Geometry: final body of the model. Coordinates: model frame, mm. A direction names the side the tool comes from. Give positions to 0.01 mm unless a question says otherwise; leave off trailing zeros. Write each loop counter-clockwise with the first axis right and the second up, starting at its lowest first coordinate (ties: lowest second). Pieces come first, ordered by that corner, then holes. Notation, with made-up numbers: (48, 62.5) - (90, 62.5) arc R19 cw to (90, 84.5) - close; hole circle Ø3 at (4, 5). An arc over 180 degrees is marked (long way). Return JSON: item names as keys, results as strings.
from build123d import *

# Parameters (mm, degrees)
SKETCH1_R                      = 11
SKETCH1_R_2                    = 1.05
BOSS_EXTRUDE1_DEPTH            = 4
SKETCH9_R                      = 6
BOSS_EXTRUDE2_DEPTH            = 15.13
SKETCH10_OUTSIDE_W             = 31.304
SKETCH10_OUTSIDE_H             = 31.304
SKETCH10_OUTSIDE_R             = 3.5
CUT_EXTRUDE2_DEPTH             = 15
FILLET1_R                      = 4.5
FILLET2_R                      = 1
FILLET4_R                      = 4
CBORE_FOR_M2_SHCS1_D           = 2.2
CBORE_FOR_M2_SHCS1_CBORE_D     = 4.4
CBORE_FOR_M2_SHCS1_CBORE_DEPTH = 2


with BuildPart() as part:
    # Sketch1 → Boss-Extrude1 (new body)
    with BuildSketch(Plane.XY):
        Circle(SKETCH1_R)
        with Locations((0, 8)):
            Circle(SKETCH1_R_2, mode=Mode.SUBTRACT)
        with Locations((8, 0)):
            Circle(SKETCH1_R_2, mode=Mode.SUBTRACT)
        with Locations((0, -8)):
            Circle(SKETCH1_R_2, mode=Mode.SUBTRACT)
    extrude(amount=BOSS_EXTRUDE1_DEPTH)

    # Sketch9 → Boss-Extrude2 (add)
    with BuildSketch(Plane(origin=(0, 0, 0), x_dir=(-1, 0, 0), z_dir=(0, 0, -1))):
        with Locations((5, 0)):
            Circle(SKETCH9_R)
    extrude(amount=BOSS_EXTRUDE2_DEPTH)

    # Sketch10 outside → Cut-Extrude2 (cut)
    with BuildSketch(Plane(origin=(0, 0, -15.13), x_dir=(-1, 0, 0), z_dir=(0, 0, -1))):
        Rectangle(SKETCH10_OUTSIDE_W, SKETCH10_OUTSIDE_H)
        with Locations((5, 0)):
            Circle(SKETCH10_OUTSIDE_R, mode=Mode.SUBTRACT)
    extrude(amount=-CUT_EXTRUDE2_DEPTH, mode=Mode.SUBTRACT)

    # Fillet1
    # the kernel refuses this fillet: 4.5 mm, written as the material it adds along each edge
    with BuildSketch(Plane(origin=(-5, 0, 0), x_dir=(-1, 0, 0), z_dir=(0, -1, 0))) as fillet1_piece_1_section:
        with BuildLine():
            CenterArc((7.073824939, 4.5), FILLET1_R, 256.19443595, 13.80556405)
            Line((6, 0.13), (6, 0))
            Line((6, 0), (7.073824939, 0))
        make_face()
    fillet1_piece_1 = revolve(axis=Axis((-5, 0, 0), (0, 0, -1)), mode=Mode.PRIVATE)
    fillet1_piece_1 = fillet1_piece_1 & Plane(origin=(0, 0, -0.023683453), x_dir=(1, 0, 0), z_dir=(0, 0, -1)) * Cylinder(11, 29, mode=Mode.PRIVATE)
    add(fillet1_piece_1)

    # Fillet2
    fillet2_edges = [part.edges().sort_by_distance(p)[0] for p in [
        (-1.5, 0, -15.13),
    ]]
    fillet(fillet2_edges, radius=FILLET2_R)

    # Fillet4
    # the kernel refuses this fillet: 4 mm, written as the material it adds along each edge
    with BuildSketch(Plane(origin=(-5, 0, -0.13), x_dir=(-1, 0, 0), z_dir=(0, -1, 0))) as fillet4_piece_1:
        with BuildLine():
            CenterArc((7.5, 3.708099244), FILLET4_R, 180, 67.975687163)
            Line((6, 0), (5.97, -0.074161985))
            ThreePointArc((5.97, -0.074161985), (4.75, -0.08), (3.5, -0.08))
            Line((3.5, -0.08), (3.42, 0))
            Line((3.42, 0), (3.42, 3.708099244))
            Line((3.42, 3.708099244), (3.5, 3.708099244))
        make_face()
    revolve(axis=Axis((-5, 0, -0.13), (0, 0, -1)))

    # CBORE for M2 SHCS1 (through all)
    with Locations(Plane(origin=(0, 0, 0), x_dir=(-1, 0, 0), z_dir=(0, 0, -1))):
        with Locations((0, 8), (-8, 0), (0, -8)):
            CounterBoreHole(CBORE_FOR_M2_SHCS1_D / 2, CBORE_FOR_M2_SHCS1_CBORE_D / 2, CBORE_FOR_M2_SHCS1_CBORE_DEPTH)


solid = part.part
Q1. Material intervals for probe 1 along Y at (x, z) = (0, 1.45); probe 2 along Y at (x, z) = (0, 3.55); probe 3 along Z at (x, y) = (-2.75, -8.5), sorted ascending. Write a range as [from, to].
Answer key:
{"probe 1": "y = [-11, -10.2], [-5.8, 5.8], [10.2, 11]", "probe 2": "y = [-11, -9.1], [-6.9, 6.9], [9.1, 11]", "probe 3": "z = [0, 4]"}
Q2. Section query D-D, the plane x = -5. Return the cut outline in (y, z), plus the area to 3 significant figures.
Answer key:
{"outline": "(-9.8, 0) - (-7.07, 0) arc R4.5 cw to (-6, -0.13) arc R4 cw to (-3.5, -3.84) - (-3.5, -14.13) arc R1 ccw to (-2.5, -15.13) - (2.5, -15.13) arc R1 ccw to (3.5, -14.13) - (3.5, -3.84) arc R4 cw to (6, -0.13) arc R4.5 cw to (7.07, 0) - (9.8, 0) - (9.8, 4) - (-9.8, 4) - close", "area": "190 mm^2"}
Q3. Section query B-B, the plane y = 8. Return the cut outline in (x, z), plus the area to 3 significant figures.
Answer key:
{"outline": "(-7.55, 0) - (-2.2, 0) - (-2.2, 2) - (-1.1, 2) - (-1.1, 4) - (-7.55, 4) - close; (1.1, 2) - (2.2, 2) - (2.2, 0) - (7.55, 0) - (7.55, 4) - (1.1, 4) - close", "area": "47.2 mm^2"}
Q4. Set-up query: faces 4 (the flat face through (0, 0, 4)), 5 (the cylindrical face through (-1.183, 9.855, 0.986)). Return all of +Z, -Z, +X, -X, +Y, -Y with unobstructed straight access to the full face (end or side cutting, diameter ignored); none if empty.
Answer key:
{"face 4": "+Z, +X, -X, +Y, -Y", "face 5": "-Z"}
Q5. Pin query (flat end, axial travel): P1, Ø1.3, axis at x = 0, y = -8, coming from the +Z side; P2, Ø3.5, axis at x = 7, y = -0.5, coming from the -Z side; P3, Ø3.5, axis at x = 0, y = 8, coming from the +Z side; P4, Ø4, axis at x = 0, y = 8, coming from the -Z side. Return the tip coordinate at first contact, or that it passes through.
Answer key:
{"P1": "passes through", "P2": "stops at z = 0", "P3": "stops at z = 4", "P4": "stops at z = 2"}
Q6. Section query C-C, the plane z = -5.75. Return the cut outline in (x, y), plus the area to 3 significant figures.
Answer key:
{"outline": "circle Ø7 at (-5, 0)", "area": "38.5 mm^2"}
Q7. Section query A-A, the plane x = 7.5. Return the cut outline in (y, z), plus the area to 3 significant figures.
Answer key:
{"outline": "(-8.05, 0) - (-2.14, 0) - (-2.14, 2) - (-0.98, 2) - (-0.98, 4) - (-8.05, 4) - close; (0.98, 2) - (2.14, 2) - (2.14, 0) - (8.05, 0) - (8.05, 4) - (0.98, 4) - close", "area": "51.9 mm^2"}
Q8. Mould query, pull axis Y, two halves, no side actions, for faces 1 (the cylindrical face through (-8.34, 1.05, -9.06)), 2 (the flat face through (3, 0, 0)), 3 (the cylindrical face through (-0.238, -9.074, 3.014)). Classes: pulls with the +Y half, pulls with the -Y half, needs draft (parallel to the pull), parting line crosses it, or undercut.
Answer key:
{"face 1": "parting line crosses it", "face 2": "needs draft", "face 3": "undercut"}
